Here's how the part is built. I have some questions about the finished solid (model axes, mm). Face numbers are marked on the shaded views. A direction names the side the tool comes from. Coordinates: 2 decimals unless noted, no trailing zeros. Order: outer loops, then holes, each group sorted by start corner. A loop starts at its lowest first (then second) coordinate and runs counter-clockwise, first axis right, second up. Notation, with made-up numbers: (67, -20) - (100, -20) arc R29 ccw to (100, 13) - close; hole circle Ø5 at (42, 44.5). An arc over 180 degrees is marked (long way). Answer in a Markdown table with one row per item. Add a question column.
Item 1: I want a section at B-B (x = 1). Please give me the cut outline in (y, z), plus the area to 3 significant figures.
Item 2: If I drill on line 1 along X through (y, z) = (10.25, 0.25); line 2 along Z through (x, y) = (4, 8.25); line 3 along Y through (x, z) = (0, -1), over which ranges is the centre line in solid material (lowest first)? Write a range as from..to.
Item 3: On a 3-axis mill with a long thin cutter (end or side, diameter ignored), from which of +Z, -Z, +X, -X, +Y, -Y can I reach the whole of each face in a straight line? I mean the marked faces 1 and 2. Say none if no direction works.
Item 4: I want a section at C-C (z = -0.75). Please give me the cut outline in (x, y), plus the area to 3 significant figures.
Item 5: Will these pins go through, and if not, where does the flat tip stop? pin 1 Ø2.5 at (x, y) = (-1.5, 8) entering from +Z; pin 2 Ø3 at (y, z) = (6, 1.5) entering from -X; pin 3 Ø1.5 at (y, z) = (6, 1) entering from +X.
Item 6: I want a section at D-D (x = -3). Please give me the cut outline in (y, z).
Item 7: I want a section at A-A (y = 6). Please give me the cut outline in (x, z).
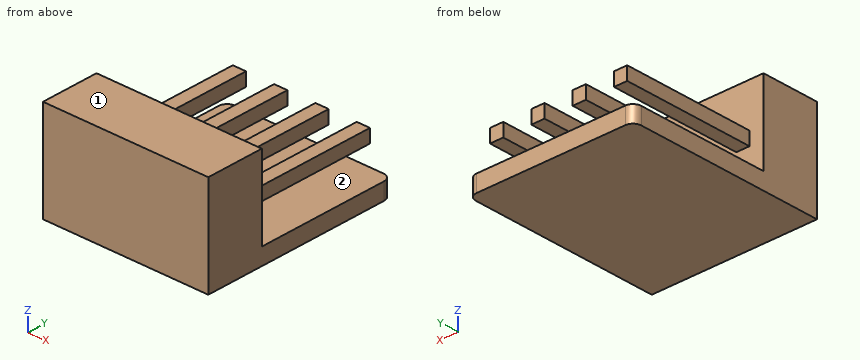
```python
from build123d import *

# Parameters (mm, degrees)
ESBO_O1_W                = 10
ESBO_O1_H                = 6.00490196
RESSALTO_EXTRUS_O1_DEPTH = 3.5
ESBO_O2_W                = 10
ESBO_O2_H                = 1
RESSALTO_EXTRUS_O2_DEPTH = 8.5
ESBO_O3_W                = 0.8
ESBO_O3_H                = 0.8
RESSALTO_EXTRUS_O3_DEPTH = 8
FILETE1_R                = 0.5


with BuildPart() as part:
    # Esboço1 → Ressalto-extrusão1 (new body)
    with BuildSketch(Plane(origin=(0, 0, 0), x_dir=(1, 0, 0), z_dir=(0, 1, 0))):
        Rectangle(ESBO_O1_W, ESBO_O1_H)
    extrude(amount=RESSALTO_EXTRUS_O1_DEPTH)

    # Esboço2 → Ressalto-extrusão2 (add)
    with BuildSketch(Plane(origin=(0, 3.5, 0), x_dir=(1, 0, 0), z_dir=(0, 1, 0))):
        with Locations((0, 2.50245098)):
            Rectangle(ESBO_O2_W, ESBO_O2_H)
    extrude(amount=RESSALTO_EXTRUS_O2_DEPTH)

    # Esboço3 → Ressalto-extrusão3 (add)
    with BuildSketch(Plane(origin=(0, 3.5, 0), x_dir=(1, 0, 0), z_dir=(0, 1, 0))):
        with Locations((-3.75, 0)):
            Rectangle(ESBO_O3_W, ESBO_O3_H)
        with Locations((-1.25, 0)):
            Rectangle(ESBO_O3_W, ESBO_O3_H)
        with Locations((1.25, 0)):
            Rectangle(ESBO_O3_W, ESBO_O3_H)
        with Locations((3.75, 0)):
            Rectangle(ESBO_O3_W, ESBO_O3_H)
    extrude(amount=RESSALTO_EXTRUS_O3_DEPTH)

    # Filete1
    filete1_edges = [part.edges().sort_by_distance(p)[0] for p in [
        (-5, 12, -2.50245098),
        (5, 12, -2.50245098),
    ]]
    fillet(filete1_edges, radius=FILETE1_R)


solid = part.part
```
Values follow:
| question | item | result |
|---|---|---|
| 1 | outline | (0, -3) - (12, -3) - (12, -2) - (3.5, -2) - (3.5, -0.4) - (11.5, -0.4) - (11.5, 0.4) - (3.5, 0.4) - (3.5, 3) - (0, 3) - close |
| 1 | area | 35.9 mm^2 |
| 2 | line 1 | x = -4.15..-3.35, -1.65..-0.85, 0.85..1.65, 3.35..4.15 |
| 2 | line 2 | z = -3..-2, -0.4..0.4 |
| 2 | line 3 | y = 0..3.5 |
| 3 | face 1 | +Z, +X, -X, +Y, -Y |
| 3 | face 2 | +X, -X, +Y |
| 4 | outline | (-5, 0) - (5, 0) - (5, 3.5) - (-5, 3.5) - close |
| 4 | area | 35.0 mm^2 |
| 5 | pin 1 | stops at z = 0.4 |
| 5 | pin 2 | stops at x = -4.15 |
| 5 | pin 3 | stops at x = 4.15 |
| 6 | outline | (0, -3) - (12, -3) - (12, -2) - (3.5, -2) - (3.5, 3) - (0, 3) - close |
| 7 | outline | (-5, -3) - (5, -3) - (5, -2) - (-5, -2) - close; (-4.15, -0.4) - (-3.35, -0.4) - (-3.35, 0.4) - (-4.15, 0.4) - close; (-1.65, -0.4) - (-0.85, -0.4) - (-0.85, 0.4) - (-1.65, 0.4) - close; (0.85, -0.4) - (1.65, -0.4) - (1.65, 0.4) - (0.85, 0.4) - close; (3.35, -0.4) - (4.15, -0.4) - (4.15, 0.4) - (3.35, 0.4) - close |
